Build history of the part. All positions in model axes, mm. Round coordinates to 2 decimals unless told otherwise and drop trailing zeros. Loops run counter-clockwise (first coordinate to the right, second up) from the corner with the lowest first, then second, coordinate; pieces in that order, holes last.
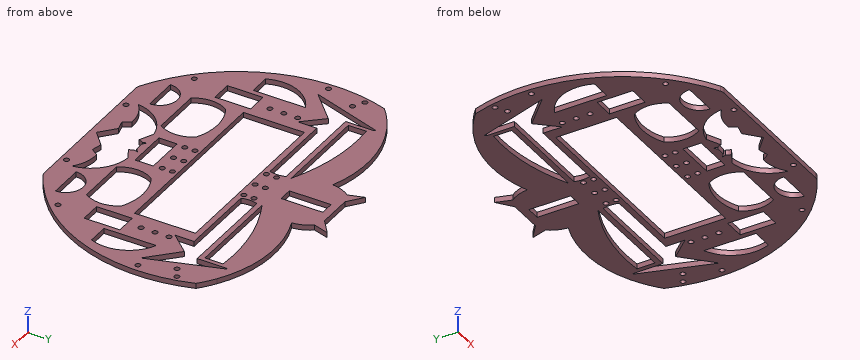
from build123d import *

# Parameters (mm, degrees)
MODEL_R                 = 1.5
MODEL_W                 = 12
MODEL_H                 = 20.5
MODEL_W_2               = 23
MODEL_H_2               = 10.5
MODEL_R_2               = 1.55
MODEL_W_3               = 105
MODEL_H_3               = 35
MODEL_W_4               = 8
MODEL_H_4               = 24
SALIENTE_EXTRUIR4_DEPTH = 3


with BuildPart() as part:
    # Model → Saliente-Extruir4 (new body)
    with BuildSketch(Plane.XY):
        with BuildLine():
            Line((-355.776015138, -60.998450132), (-267.599829389, -60.998450132))
            ThreePointArc((-267.599829389, -60.998450132), (-266.347451458, -60.839064712), (-265.17491784, -60.371069939))
            ThreePointArc((-265.17491784, -60.371069939), (-222.293639907, -11.236587904), (-220.746441381, 53.960095284))
            ThreePointArc((-220.746441381, 53.960095284), (-225.084945906, 57.549539585), (-229.703657645, 60.770445324))
            ThreePointArc((-229.703657645, 60.770445324), (-259.877190608, 71.193554512), (-291.497465301, 66.807038251))
            ThreePointArc((-291.497465301, 66.807038251), (-292.755686274, 72.473376479), (-295.600352839, 77.532860749))
            Line((-295.600352839, 77.532860749), (-295.591792135, 77.56086155))
            Line((-295.591792135, 77.56086155), (-292.895401724, 86.380357187))
            Line((-292.895401724, 86.380357187), (-301.389427163, 79.7440972))
            Line((-301.389427163, 79.7440972), (-311.281389026, 79.7440972))
            Line((-311.281389026, 79.7440972), (-321.173350888, 79.7440972))
            Line((-321.173350888, 79.7440972), (-329.667376328, 86.380357187))
            Line((-329.667376328, 86.380357187), (-326.970985917, 77.56086155))
            Line((-326.970985917, 77.56086155), (-326.962425213, 77.532860749))
            ThreePointArc((-326.962425213, 77.532860749), (-329.807091778, 72.473376479), (-331.06531275, 66.807038251))
            ThreePointArc((-331.06531275, 66.807038251), (-363.187871913, 71.263043057), (-393.802821484, 60.565396182))
            ThreePointArc((-393.802821484, 60.565396182), (-398.392570042, 57.331333816), (-402.704441803, 53.735125656))
            ThreePointArc((-402.704441803, 53.735125656), (-401.039186713, -11.347086765), (-358.200926687, -60.371069939))
            ThreePointArc((-358.200926687, -60.371069939), (-357.028393069, -60.839064712), (-355.776015138, -60.998450132))
        make_face()
        with Locations((-377.655085345, -40.498450132)):
            Circle(MODEL_R, mode=Mode.SUBTRACT)
        with Locations((-340.371601562, -57.498450132)):
            Circle(MODEL_R, mode=Mode.SUBTRACT)
        with BuildLine():
            Line((-347.094522431, -47.905049404), (-367.094522431, -47.905049404))
            ThreePointArc((-367.094522431, -47.905049404), (-357.094522431, -37.905049404), (-347.094522431, -47.905049404))
        make_face(mode=Mode.SUBTRACT)
        with Locations((-374.687922263, -13.08422583)):
            Rectangle(MODEL_W, MODEL_H, mode=Mode.SUBTRACT)
        with BuildLine():
            Line((-383.564259156, 19.787814732), (-383.564259156, -10.212185268))
            Line((-383.564259156, -10.212185268), (-395.564259156, -10.212185268))
            ThreePointArc((-395.564259156, -10.212185268), (-395.74209606, 7.258949494), (-383.564259156, 19.787814732))
        make_face(mode=Mode.SUBTRACT)
        with Locations((-373.687922263, 5.251549869)):
            Circle(MODEL_R, mode=Mode.SUBTRACT)
        with BuildLine():
            ThreePointArc((-333.187901103, -13.08422583), (-330.056215503, -23.08422583), (-333.187901103, -33.08422583))
            Line((-333.187901103, -33.08422583), (-361.987901103, -33.08422583))
            ThreePointArc((-361.987901103, -33.08422583), (-365.119586704, -23.08422583), (-361.987901103, -13.08422583))
            ThreePointArc((-361.987901103, -13.08422583), (-347.587901103, -9.377791016), (-333.187901103, -13.08422583))
        make_face(mode=Mode.SUBTRACT)
        with Locations((-322.48953205, -13.098450131)):
            Circle(MODEL_R, mode=Mode.SUBTRACT)
        with Locations((-322.48953205, -7.248450131)):
            Circle(MODEL_R, mode=Mode.SUBTRACT)
        with BuildLine():
            ThreePointArc((-307.724846888, -33.315800094), (-307.00591302, -34.594485844), (-306.687922263, -36.02654207))
            Line((-306.687922263, -36.02654207), (-299.934718732, -32.331670932))
            ThreePointArc((-299.934718732, -32.331670932), (-286.208260503, -38.793667419), (-279.594522431, -52.447660346))
            ThreePointArc((-279.594522431, -52.447660346), (-286.59107666, -48.299677368), (-294.638759456, -47.119704707))
            Line((-294.638759456, -47.119704707), (-297.434723974, -51.26489257))
            Line((-297.434723974, -51.26489257), (-303.256498331, -49.813361196))
            Line((-303.256498331, -49.813361196), (-311.687922263, -57.405049404))
            Line((-311.687922263, -57.405049404), (-320.180334417, -49.881622626))
            Line((-320.180334417, -49.881622626), (-326.002108775, -51.333154))
            Line((-326.002108775, -51.333154), (-328.798073292, -47.187966137))
            ThreePointArc((-328.798073292, -47.187966137), (-336.771965329, -48.364327922), (-343.72129462, -52.447660346))
            ThreePointArc((-343.72129462, -52.447660346), (-337.595412912, -39.178561893), (-324.720148301, -32.263147106))
            Line((-324.720148301, -32.263147106), (-316.687922263, -36.02654207))
            ThreePointArc((-316.687922263, -36.02654207), (-316.369931507, -34.594485844), (-315.650997638, -33.315800094))
            Line((-315.650997638, -33.315800094), (-316.334621158, -31.079768314))
            Line((-316.334621158, -31.079768314), (-314.187922263, -32.756953305))
            Line((-314.187922263, -32.756953305), (-309.187922263, -32.756953305))
            Line((-309.187922263, -32.756953305), (-307.041223368, -31.079768314))
            Line((-307.041223368, -31.079768314), (-307.724846888, -33.315800094))
        make_face(mode=Mode.SUBTRACT)
        with Locations((-283.004001562, -57.498450132)):
            Circle(MODEL_R, mode=Mode.SUBTRACT)
        with BuildLine():
            ThreePointArc((-276.281322096, -47.905049404), (-266.281322096, -37.905049404), (-256.281322096, -47.905049404))
            Line((-256.281322096, -47.905049404), (-276.281322096, -47.905049404))
        make_face(mode=Mode.SUBTRACT)
        with Locations((-246.258954343, -40.498450132)):
            Circle(MODEL_R, mode=Mode.SUBTRACT)
        with Locations((-311.687922263, -23.155049404)):
            Rectangle(MODEL_W_2, MODEL_H_2, mode=Mode.SUBTRACT)
        with Locations((-311.687922263, -13.098450131)):
            Circle(MODEL_R, mode=Mode.SUBTRACT)
        with Locations((-300.790542177, -13.098450131)):
            Circle(MODEL_R, mode=Mode.SUBTRACT)
        with Locations((-311.687922263, -7.248450131)):
            Circle(MODEL_R, mode=Mode.SUBTRACT)
        with Locations((-300.790542177, -7.248450131)):
            Circle(MODEL_R, mode=Mode.SUBTRACT)
        with BuildLine():
            ThreePointArc((-261.387922263, -13.08422583), (-258.256236663, -23.08422583), (-261.387922263, -33.08422583))
            Line((-261.387922263, -33.08422583), (-290.187922263, -33.08422583))
            ThreePointArc((-290.187922263, -33.08422583), (-293.319607864, -23.08422583), (-290.187922263, -13.08422583))
            ThreePointArc((-290.187922263, -13.08422583), (-275.787922263, -9.377788158), (-261.387922263, -13.08422583))
        make_face(mode=Mode.SUBTRACT)
        with Locations((-248.687922263, -13.08422583)):
            Rectangle(MODEL_W, MODEL_H, mode=Mode.SUBTRACT)
        with Locations((-249.687922263, 5.251549869)):
            Circle(MODEL_R_2, mode=Mode.SUBTRACT)
        with BuildLine():
            Line((-227.811585371, -10.212185268), (-239.811585371, -10.212185268))
            Line((-239.811585371, -10.212185268), (-239.811585371, 19.787814732))
            ThreePointArc((-239.811585371, 19.787814732), (-227.633748467, 7.258949494), (-227.811585371, -10.212185268))
        make_face(mode=Mode.SUBTRACT)
        with Locations((-403.839630577, 21.001549869)):
            Circle(MODEL_R, mode=Mode.SUBTRACT)
        with Locations((-373.687922263, 13.251549869)):
            Circle(MODEL_R, mode=Mode.SUBTRACT)
        with Locations((-373.687922263, 21.251549869)):
            Circle(MODEL_R, mode=Mode.SUBTRACT)
        with Locations((-396.445915559, 39.162490233)):
            Circle(MODEL_R, mode=Mode.SUBTRACT)
        with Locations((-402.508093385, 42.662490233)):
            Circle(MODEL_R, mode=Mode.SUBTRACT)
        with BuildLine():
            ThreePointArc((-325.594522431, 43.223476573), (-324.856684533, 38.624455287), (-325.594522431, 34.025434))
            Line((-325.594522431, 34.025434), (-336.444815564, 34.053135683))
            Line((-336.444815564, 34.053135683), (-370.619106993, 34.053135683))
            Line((-370.619106993, 34.053135683), (-370.619106993, 23.0817416))
            Line((-370.619106993, 23.0817416), (-380.871401066, 34.540754549))
            Line((-380.871401066, 34.540754549), (-396.971212692, 18.93698732))
            Line((-396.971212692, 18.93698732), (-383.824116508, 59.975759861))
            Line((-383.824116508, 59.975759861), (-383.063023773, 59.125084739))
            Line((-383.063023773, 59.125084739), (-383.036780558, 43.223476573))
            Line((-383.036780558, 43.223476573), (-325.594522431, 43.223476573))
        make_face(mode=Mode.SUBTRACT)
        with Locations((-322.48953205, 33.751530494)):
            Circle(MODEL_R, mode=Mode.SUBTRACT)
        with Locations((-322.48953205, 39.601530494)):
            Circle(MODEL_R, mode=Mode.SUBTRACT)
        with BuildLine():
            Line((-325.594522431, 46.179790486), (-380.702976272, 46.117817898))
            Line((-380.702976272, 46.117817898), (-380.811334061, 56.516231765))
            ThreePointArc((-380.811334061, 56.516231765), (-352.478131532, 55.219843079), (-325.594522431, 46.179790486))
        make_face(mode=Mode.SUBTRACT)
        with Locations((-311.687922263, 13.251549869)):
            Rectangle(MODEL_W_3, MODEL_H_3, mode=Mode.SUBTRACT)
        with Locations((-311.687922263, 33.751530494)):
            Circle(MODEL_R, mode=Mode.SUBTRACT)
        with Locations((-300.790542177, 33.751530494)):
            Circle(MODEL_R, mode=Mode.SUBTRACT)
        with Locations((-311.687922263, 39.601530494)):
            Circle(MODEL_R, mode=Mode.SUBTRACT)
        with Locations((-300.790542177, 39.601530494)):
            Circle(MODEL_R, mode=Mode.SUBTRACT)
        with Locations((-249.687922263, 13.251549869)):
            Circle(MODEL_R, mode=Mode.SUBTRACT)
        with Locations((-249.687922263, 21.251549869)):
            Circle(MODEL_R_2, mode=Mode.SUBTRACT)
        with Locations((-220.074429493, 21.001549869)):
            Circle(MODEL_R, mode=Mode.SUBTRACT)
        with BuildLine():
            Line((-297.567305128, 43.199876989), (-240.144576222, 43.103241367))
            Line((-240.144576222, 43.103241367), (-240.088099797, 60.046643019))
            Line((-240.088099797, 60.046643019), (-239.588301513, 60.668146026))
            Line((-239.588301513, 60.668146026), (-226.251035034, 18.793336547))
            Line((-226.251035034, 18.793336547), (-242.324564615, 34.424175709))
            Line((-242.324564615, 34.424175709), (-252.596128298, 22.982432354))
            Line((-252.596128298, 22.982432354), (-252.577664773, 33.953810901))
            Line((-252.577664773, 33.953810901), (-286.751907811, 34.011322086))
            Line((-286.751907811, 34.011322086), (-297.602232198, 34.00188017))
            ThreePointArc((-297.602232198, 34.00188017), (-298.323089741, 38.603682167), (-297.567305128, 43.199876989))
        make_face(mode=Mode.SUBTRACT)
        with Locations((-227.197722974, 39.275050872)):
            Circle(MODEL_R, mode=Mode.SUBTRACT)
        with Locations((-221.135545147, 42.775050872)):
            Circle(MODEL_R, mode=Mode.SUBTRACT)
        with Locations((-311.488157346, 63.138374517)):
            Rectangle(MODEL_W_4, MODEL_H_4, mode=Mode.SUBTRACT)
        with BuildLine():
            Line((-242.564510466, 56.516231765), (-242.672868255, 46.117817898))
            Line((-242.672868255, 46.117817898), (-297.567305128, 46.179790486))
            ThreePointArc((-297.567305128, 46.179790486), (-270.794233717, 55.223615887), (-242.564510466, 56.516231765))
        make_face(mode=Mode.SUBTRACT)
    extrude(amount=SALIENTE_EXTRUIR4_DEPTH)


solid = part.part
(1) Probe line 1 (Y direction, x = -309, z = 1.85); line 2 (X direction, y = -19.5, z = 1.2); line 3 (Y direction, x = -279.5, z = 1.95). List the from-to ranges inside material, lowest first.
Responses:
line 1: y = -61 to -54.98, -32.61 to -28.41, -17.91 to -4.25, 30.75 to 51.14, 75.14 to 79.74
line 2: x = -397.41 to -380.69, -368.69 to -364.75, -330.43 to -323.19, -300.19 to -292.95, -258.63 to -254.69, -242.69 to -225.96
line 3: y = -61 to -33.08, -9.61 to -4.25, 30.75 to 34, 43.17 to 46.16, 53.19 to 70.28
(2) Slice it at A-A on y = -20. List the corners of the cut face in (x, z).
Responses:
outline: (-397.16, 0) - (-380.69, 0) - (-380.69, 3) - (-397.16, 3) - close; (-368.69, 0) - (-364.85, 0) - (-364.85, 3) - (-368.69, 3) - close; (-330.33, 0) - (-323.19, 0) - (-323.19, 3) - (-330.33, 3) - close; (-300.19, 0) - (-293.05, 0) - (-293.05, 3) - (-300.19, 3) - close; (-258.53, 0) - (-254.69, 0) - (-254.69, 3) - (-258.53, 3) - close; (-242.69, 0) - (-226.21, 0) - (-226.21, 3) - (-242.69, 3) - close
(3) Slice it at B-B on z = 2.2. Count the separate pieces of the cut face and the enclosed holes in it, plus the area to 3 significant figures.
Responses:
separate pieces: 1
enclosed holes: 44
area: 11,800 mm2
(4) Pin check, flat tips, straight feed: P1, Ø1.5, axis at x = -312.5, z = 2, coming from the +Y side; P2, Ø1.5, axis at y = 62.5, z = 1.5, coming from the -X side; P3, Ø0.9, axis at x = -375, z = 2, coming from the -Y side. Stop position of each tip, or through.
Responses:
P1: stops at y = 79.74
P2: stops at x = -391.9
P3: stops at y = -48.93
